Design review of the part built by this model. Coordinates are the model's own, in mm. Face numbers are marked on the shaded views. A direction names the side the tool comes from. Coordinates: 2 decimals unless noted, no trailing zeros. Loops run counter-clockwise (first coordinate to the right, second up) from the corner with the lowest first, then second, coordinate; pieces in that order, holes last. Notation, with made-up numbers: (49.5, -36) - (70.5, -36) arc R28 ccw to (70.5, -9) - close; hole circle Ø7 at (7.5, 28.5). An arc over 180 degrees is marked (long way). One line per question, with ' | ' between items.
from build123d import *

# Parameters (mm, degrees)
F3_R      = 54
F4_DEPTH  = 10
F5_R      = 4.99999
F7_DEPTH  = 5
F8_R      = 37.5
F9_DEPTH  = 37.5
F11_R     = 10
F12_DEPTH = 10
F13_R     = 10
F14_DEPTH = 10
F15_R     = 6
F16_DEPTH = 2


# Not quite as in the source:
# - a fillet or chamfer is up to 0.001 mm smaller than in the source, because OpenCascade refuses the exact size


with BuildPart() as f2:
    # F1 (on Front) → F2 (revolve)
    with BuildSketch(Plane.XZ):
        with BuildLine():
            Line((0, 820), (0, 0))
            Line((0, 0), (195, 0))
            Line((195, 0), (195, 770))
            ThreePointArc((195, 770), (180.3553390593, 805.3553390593), (145, 820))
            Line((145, 820), (0, 820))
        make_face()
    revolve(axis=Axis((0, 0, 410), (0, 0, -1)))

    # F3 (on face) → F4 (cut)
    with BuildSketch(Plane.XY.offset(820)):
        Circle(F3_R)
    extrude(amount=-F4_DEPTH, mode=Mode.SUBTRACT)

    # F5 (radius 5 in the source; OpenCascade refuses exactly that, so slightly less here)
    f5_edges = [f2.edges().sort_by_distance(p)[0] for p in [
        (-54, 0, 820),
        (-54, 0, 810),
    ]]
    fillet(f5_edges, radius=F5_R)

    # F6 (on face) → F7 (join)
    with BuildSketch(Plane.XY.offset(810)):
        Polygon((-17.6040764009, -42.5), (17.6040764009, -42.5), (42.5, -17.6040764009), (42.5, 17.6040764009), (17.6040764009, 42.5), (-17.6040764009, 42.5), (-42.5, 17.6040764009), (-42.5, -17.6040764009), align=None)
    extrude(amount=F7_DEPTH)

    # F8 (on face) → F9 (join, symmetric)
    with BuildSketch(Plane.XY.offset(820)):
        Circle(F8_R)
    extrude(amount=F9_DEPTH, both=True)

    # F11 (on offset) → F12 (cut)
    with BuildSketch(Plane.XZ.offset(195)):
        with Locations((0, 175)):
            Circle(F11_R)
        with Locations((0, 257)):
            Circle(F11_R)
        with Locations((0, 333)):
            Circle(F11_R)
        with Locations((0, 412)):
            Circle(F11_R)
        with Locations((0, 493)):
            Circle(F11_R)
        with Locations((0, 573)):
            Circle(F11_R)
    extrude(amount=-F12_DEPTH, mode=Mode.SUBTRACT)

    # F13 (on face) → F14 (cut)
    with BuildSketch(Plane.XY.offset(820)):
        with Locations((0, -130)):
            Circle(F13_R)
    extrude(amount=-F14_DEPTH, mode=Mode.SUBTRACT)

    # F15 (on face) → F16 (join)
    with BuildSketch(Plane(origin=(0, 0, 0), x_dir=(1, 0, 0), z_dir=(0, 0, -1))):
        with BuildLine():
            ThreePointArc((-153.7957249081, 178.5444622496), (-160.8667927199, 181.4733944377), (-167.9378605318, 178.5444622496))
            Line((-167.9378605318, 178.5444622496), (-178.5444622496, 167.9378605318))
            ThreePointArc((-178.5444622496, 167.9378605318), (-181.4733944377, 160.8667927199), (-178.5444622496, 153.7957249081))
            Line((-178.5444622496, 153.7957249081), (-146.1599508606, 121.411213519))
            Line((-146.1599508606, 121.411213519), (-121.411213519, 146.1599508606))
            Line((-121.411213519, 146.1599508606), (-153.7957249081, 178.5444622496))
        make_face()
        with Locations((-156.4564352241, 156.4564352241)):
            Circle(F15_R, mode=Mode.SUBTRACT)
        with BuildLine():
            Line((-153.7957249081, -178.5444622496), (-121.411213519, -146.1599508606))
            Line((-121.411213519, -146.1599508606), (-146.1599508606, -121.411213519))
            Line((-146.1599508606, -121.411213519), (-178.5444622496, -153.7957249081))
            ThreePointArc((-178.5444622496, -153.7957249081), (-181.4733944377, -160.8667927199), (-178.5444622496, -167.9378605318))
            Line((-178.5444622496, -167.9378605318), (-167.9378605318, -178.5444622496))
            ThreePointArc((-167.9378605318, -178.5444622496), (-160.8667927199, -181.4733944377), (-153.7957249081, -178.5444622496))
        make_face()
        with Locations((-156.4564352241, -156.4564352241)):
            Circle(F15_R, mode=Mode.SUBTRACT)
        with BuildLine():
            Line((178.5444622496, -153.7957249081), (146.1599508606, -121.411213519))
            Line((146.1599508606, -121.411213519), (121.411213519, -146.1599508606))
            Line((121.411213519, -146.1599508606), (153.7957249081, -178.5444622496))
            ThreePointArc((153.7957249081, -178.5444622496), (160.8667927199, -181.4733944377), (167.9378605318, -178.5444622496))
            Line((167.9378605318, -178.5444622496), (178.5444622496, -167.9378605318))
            ThreePointArc((178.5444622496, -167.9378605318), (181.4733944377, -160.8667927199), (178.5444622496, -153.7957249081))
        make_face()
        with Locations((156.4564352241, -156.4564352241)):
            Circle(F15_R, mode=Mode.SUBTRACT)
        with BuildLine():
            Line((153.7957249081, 178.5444622496), (121.411213519, 146.1599508606))
            Line((121.411213519, 146.1599508606), (146.1599508606, 121.411213519))
            Line((146.1599508606, 121.411213519), (178.5444622496, 153.7957249081))
            ThreePointArc((178.5444622496, 153.7957249081), (181.4733944377, 160.8667927199), (178.5444622496, 167.9378605318))
            Line((178.5444622496, 167.9378605318), (167.9378605318, 178.5444622496))
            ThreePointArc((167.9378605318, 178.5444622496), (160.8667927199, 181.4733944377), (153.7957249081, 178.5444622496))
        make_face()
        with Locations((156.4564352241, 156.4564352241)):
            Circle(F15_R, mode=Mode.SUBTRACT)
    extrude(amount=-F16_DEPTH)


solid = f2.part
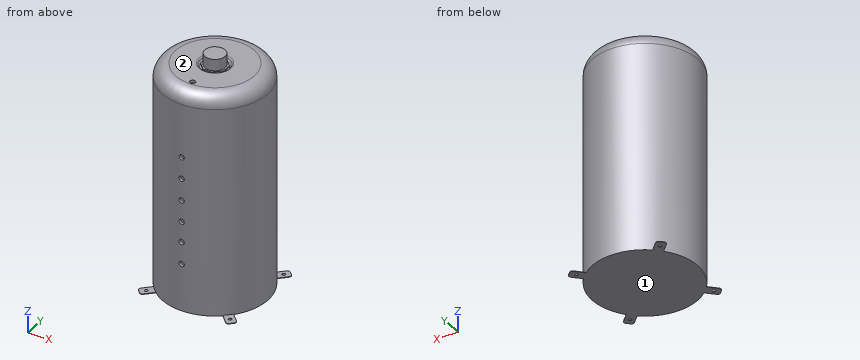
Q1. Take a section at A-A (z = 548). Give the boundary of the cut face in (x, y).
Returned:
outline: circle Ø390 at (0, 0)
Q2. Take a section at B-B (z = 257). Give the boundary of the cut face in (x, y).
Returned:
outline: (-10, -194.74) - (-10, -185) - (10, -185) - (10, -194.74) arc R195 ccw (long way) to start
Q3. Tool access review of the marked faces 1 and 2: name each direction out of +Z, -Z, +X, -X, +Y, -Y from which nothing blocks a thin tool from reaching the whole face with its end or side.
Returned:
face 1: -Z, +X, -X, +Y, -Y | face 2: +Z
Q4. For pin 1 (4 mm diameter, centred on y = 110.5, z = 440, fed in from +X); pin 2 (1.5 mm diameter, centred on x = 96.5, z = 130, fed in from -Y); pin 3 (6 mm diameter, centred on y = 24, z = 185, fed in from +X), all flat-tipped, find the tip position at first contact; note any pin that passes through.
Returned:
pin 1: stops at x = 162.03 | pin 2: stops at y = -169.87 | pin 3: stops at x = 193.87
Q5. To check wall thickness, follow line 1 along Z through (x, y) = (80.5, 77); line 2 along Y through (x, z) = (125, 268); line 3 along Y through (x, z) = (-0.5, 143). State the ranges of each line that lie inside material, in increasing order.
Returned:
line 1: z = 0 to 820 | line 2: y = -149.67 to 149.67 | line 3: y = -195 to 195
